The model under review builds one solid part; all positions refer to its coordinate system, in mm. Face numbers are marked on the shaded views. Give positions to 0.01 mm unless a question says otherwise; leave off trailing zeros. Loops run counter-clockwise (first coordinate to the right, second up) from the corner with the lowest first, then second, coordinate; pieces in that order, holes last. Notation, with made-up numbers: M 1,84 L 11,84 A19 ccw 11,116 Z; hole C -22,22.25 d8. An arc over 180 degrees is marked long. Return JSON: item names as keys, results as strings.
```python
from build123d import *

# Parameters (mm, degrees)
SKETCH1_R           = 1.55
BOSS_EXTRUDE1_DEPTH = 7
FILLET1_R           = 0.2


with BuildPart() as part:
    # Sketch1 → Boss-Extrude1 (new body)
    with BuildSketch(Plane(origin=(0, 0, 0), x_dir=(1, 0, 0), z_dir=(0, 1, 0))):
        Polygon((3.897114317, 4.5), (1.299038106, 4.5), (0, 2.25), (1.299038106, 0), (3.897114317, 0), (5.196152423, 2.25), align=None)
        with Locations(Location((2.598076211, 2.25, 0), (0, 0, 270))):
            Circle(SKETCH1_R, mode=Mode.SUBTRACT)
    extrude(amount=BOSS_EXTRUDE1_DEPTH)

    # Fillet1
    fillet1_edges = [part.edges().sort_by_distance(p)[0] for p in [
        (0.649519053, 0, -1.125),
        (0.649519053, 0, -3.375),
        (2.598076211, 0, -4.5),
        (2.598076211, 0, -3.8),
        (2.598076211, 7, -4.5),
        (3.897114317, 3.5, -4.5),
        (5.196152423, 3.5, -2.25),
        (3.897114317, 3.5, 0),
        (1.299038106, 3.5, 0),
        (0, 3.5, -2.25),
        (1.299038106, 3.5, -4.5),
        (0.649519053, 7, -3.375),
        (0.649519053, 7, -1.125),
        (2.598076211, 7, 0),
        (4.54663337, 7, -1.125),
        (4.54663337, 7, -3.375),
        (2.598076211, 7, -3.8),
        (4.54663337, 0, -3.375),
        (4.54663337, 0, -1.125),
        (2.598076211, 0, 0),
    ]]
    fillet(fillet1_edges, radius=FILLET1_R)


solid = part.part
```
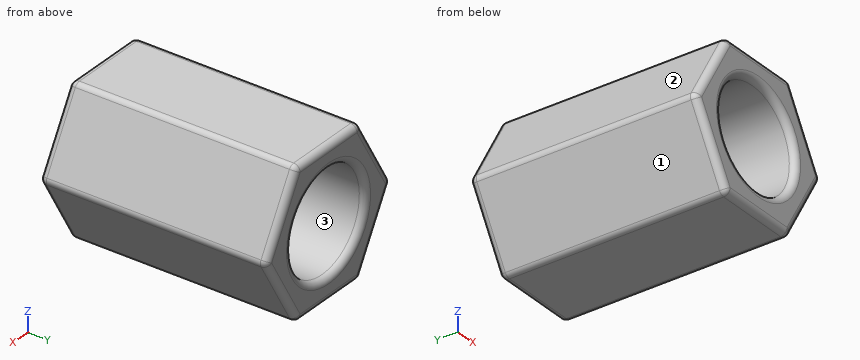
1) The part is to be moulded in two halves that separate along Z. For the marked faces 1, 2 and 3, say which applies: released by +Z, released by -Z, zero draft, split by the parting line, or undercut.
From the geometry:
{"face 1": "released by -Z", "face 2": "released by +Z", "face 3": "undercut"}
2) Consider section A-A on y = 6.25. Write out the cut boundary in (x, z).
From the geometry:
{"outline": "M 0.06,-2.35 L 1.24,-4.4 A0.2 ccw 1.41,-4.5 L 3.78,-4.5 A0.2 ccw 3.95,-4.4 L 5.14,-2.35 A0.2 ccw 5.14,-2.15 L 3.95,-0.1 A0.2 ccw 3.78,0 L 1.41,0 A0.2 ccw 1.24,-0.1 L 0.06,-2.15 A0.2 ccw Z; hole C 2.6,-2.25 d3.1"}
3) Wall thickness on L1, parallel to X at y = 3, z = -2.25; L2, parallel to Z at x = 2.3, y = 1; L3, parallel to Z at x = 3.3, y = 1.5: over which ranges is each line inside the solid? List them lowest first. Write a range as from..to.
From the geometry:
{"L1": "0.03..1.05, 4.15..5.17", "L2": "-4.5..-3.77, -0.73..0", "L3": "-4.5..-3.63, -0.87..0"}
